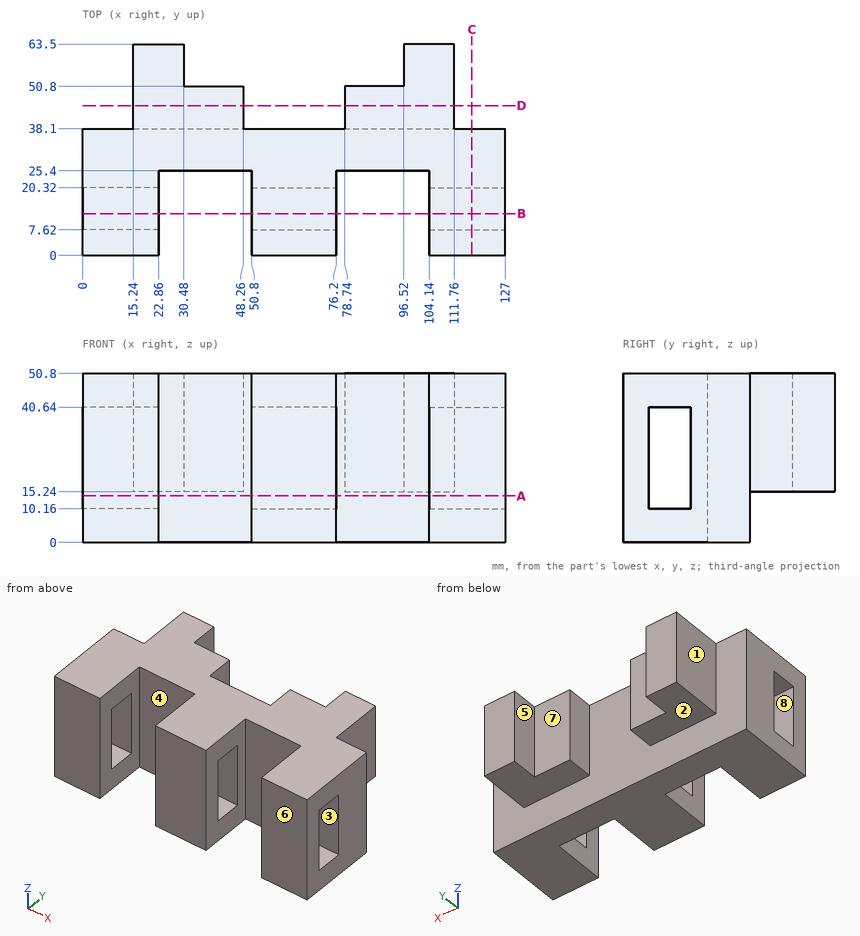
Here's the drawing with two shaded views (mm, measured from the low corner). I have some questions. A direction names the side the tool comes from. Give positions to 0.01 mm unless a question says otherwise; leave off trailing zeros. Order: outer loops, then holes, each group sorted by start corner. A loop starts at its lowest first (then second) coordinate and runs counter-clockwise, first axis right, second up.
Q1. Suppose I cut it at A-A, the plane z = 14. Write out the boundary of the cut face in (x, y), and give its area (3 significant figures).
Q2. I'm going to push flat-ended pins straight in: P1, Ø1, axis at x = 112, y = 54.5, coming from the -Z side; P2, Ø6.5, axis at y = 59, z = 29.5, coming from the -X side; P3, Ø5.5, axis at x = 43, z = 28.5, coming from the +Y side. Where does each tip first touch, or does it pass through?
Q3. Suppose I cut it at D-D, the plane y = 45. Write out the boundary of the cut face in (x, z).
Q4. We'd pull the mould along Y, two halves only. Please class the marked faces 6, 7 and 8: +Y half, -Y half, draft (parallel to the pull), parting line (faces both ways), or undercut.
Q5. If I drill on line 1 along X through (y, z) = (21, 43.5); line 2 along Y through (x, z) = (68.5, 25); line 3 along Z through (x, y) = (113, 13.5), over which ranges is the centre line in solid material (lowest first)?
Q6. For the marked faces 1, 2, 3, 4 and 5, which set-ups out of +Z, -Z, +X, -X, +Y, -Y let a thin tool reach every point of the face, with its end or its side?
Q7. Suppose I cut it at C-C, the plane x = 117. Write out the boundary of the cut face in (y, z), and give its area (3 significant figures).
Q8. Suppose I cut it at B-B, the plane y = 12.5. Write out the boundary of the cut face in (x, z), and give its area (3 significant figures).
Solution:
1. outline: (0, 0) - (22.86, 0) - (22.86, 7.62) - (0, 7.62) - close; (0, 20.32) - (22.86, 20.32) - (22.86, 25.4) - (50.8, 25.4) - (50.8, 20.32) - (76.2, 20.32) - (76.2, 25.4) - (104.14, 25.4) - (104.14, 20.32) - (127, 20.32) - (127, 38.1) - (0, 38.1) - close; (50.8, 0) - (76.2, 0) - (76.2, 7.62) - (50.8, 7.62) - close; (104.14, 0) - (127, 0) - (127, 7.62) - (104.14, 7.62) - close
1. area: 2,520 mm2
2. P1: stops at z = 15.24
2. P2: stops at x = 15.24
2. P3: stops at y = 50.8
3. outline: (15.24, 15.24) - (48.26, 15.24) - (48.26, 50.8) - (15.24, 50.8) - close; (78.74, 15.24) - (111.76, 15.24) - (111.76, 50.8) - (78.74, 50.8) - close
4. face 6: -Y half
4. face 7: +Y half
4. face 8: undercut
5. line 1: x = 0 to 22.86, 50.8 to 76.2, 104.14 to 127
5. line 2: y = 0 to 7.62, 20.32 to 38.1
5. line 3: z = 0 to 10.16, 40.64 to 50.8
6. face 1: +Z, -Z, -X, +Y
6. face 2: -Z, +X, -X, +Y
6. face 3: +X, -X
6. face 4: +Z, -Z, -Y
6. face 5: +Z, -Z, +Y
7. outline: (0, 0) - (38.1, 0) - (38.1, 50.8) - (0, 50.8) - close; hole (7.62, 10.16) - (20.32, 10.16) - (20.32, 40.64) - (7.62, 40.64) - close
7. area: 1,550 mm2
8. outline: (0, 0) - (22.86, 0) - (22.86, 10.16) - (0, 10.16) - close; (0, 40.64) - (22.86, 40.64) - (22.86, 50.8) - (0, 50.8) - close; (50.8, 0) - (76.2, 0) - (76.2, 10.16) - (50.8, 10.16) - close; (50.8, 40.64) - (76.2, 40.64) - (76.2, 50.8) - (50.8, 50.8) - close; (104.14, 0) - (127, 0) - (127, 10.16) - (104.14, 10.16) - close; (104.14, 40.64) - (127, 40.64) - (127, 50.8) - (104.14, 50.8) - close
8. area: 1,450 mm2
